from build123d import *

# Parameters (mm, degrees)
CROQUIS1_W              = 10
CROQUIS1_H              = 12.25
SALIENTE_EXTRUIR1_DEPTH = 6.5
CROQUIS3_R              = 1
CROQUIS3_W              = 12.25
CROQUIS3_H              = 3.5
CORTAR_EXTRUIR1_DEPTH   = 35.4


with BuildPart() as part:
    # Croquis1 → Saliente-Extruir1 (new body)
    with BuildSketch(Plane(origin=(0, 0, 0), x_dir=(1, 0, 0), z_dir=(0, 1, 0))):
        Polygon((-15.606807411, 13.619327476), (-15.606807411, 6.744327476), (-9.43180722, 6.744327476), (-9.43180722, -5.505672524), (-15.606807411, -5.505672524), (-15.606807411, -12.380672524), (17.093193352, -12.380672524), (17.093193352, -5.505672524), (10.918193161, -5.505672524), (10.918193161, 6.744327476), (17.093193352, 6.744327476), (17.093193352, 13.619327476), align=None)
        with Locations((0.743192971, 0.619327476)):
            Rectangle(CROQUIS1_W, CROQUIS1_H, mode=Mode.SUBTRACT)
    extrude(amount=SALIENTE_EXTRUIR1_DEPTH)

    # Croquis3 → Cortar-Extruir1 (cut)
    with BuildSketch(Plane.ZY.offset(15.606807411)):
        with Locations((-10.181827476, 3.25)):
            Circle(CROQUIS3_R)
        with Locations((8.943172524, 3.25)):
            Circle(CROQUIS3_R)
        with Locations((-0.619327476, 4.75)):
            Rectangle(CROQUIS3_W, CROQUIS3_H)
    extrude(amount=-CORTAR_EXTRUIR1_DEPTH, mode=Mode.SUBTRACT)


solid = part.part
CAD build for the part. Positions are in the model's coordinates, mm. A direction names the side the tool comes from. Give positions to 0.01 mm unless a question says otherwise; leave off trailing zeros. Write each loop counter-clockwise with the first axis right and the second up, starting at its lowest first coordinate (ties: lowest second). Pieces come first, ordered by that corner, then holes. Notation, with made-up numbers: (65, 3) -> (89, 3) arc R15 cw to (89, 21) -> close; hole circle Ø9 at (81.25, 71.5). An arc over 180 degrees is marked (long way). Return JSON: item names as keys, results as strings.
Item 1: Tool access for faces 5 (the flat face through (5.743, 1, -1)), 6 (the flat face through (1, 3, -6.744)), 7 (the flat face through (-7, 3, -1)), 8 (the flat face through (10.918, 1, -1)), 9 (the flat face through (-9.432, 1, -1)): list every direction of +Z, -Z, +X, -X, +Y, -Y with a clear straight run to the whole face (end or side of a thin tool).
Answer below:
{"face 5": "+Y, -Y", "face 6": "+Y", "face 7": "+X, -X, +Y", "face 8": "+X, +Y, -Y", "face 9": "-X, +Y, -Y"}
Item 2: Band-saw the part on A-A (x = 0.5). List the corners of the cut face in (y, z).
Answer below:
{"outline": "(0, -13.62) -> (6.5, -13.62) -> (6.5, -6.74) -> (0, -6.74) -> close; (0, 5.51) -> (6.5, 5.51) -> (6.5, 12.38) -> (0, 12.38) -> close; hole circle Ø2 at (3.25, -10.18); hole circle Ø2 at (3.25, 8.94)"}
Item 3: Drop flat-ended pins along their axis: pin 1 (2.5 mm diameter, centred on x = -7, z = -3, fed in from +Y); pin 2 (1.5 mm diameter, centred on y = 1, z = -3, fed in from +X); pin 3 (0.9 mm diameter, centred on y = 2, z = -0.5, fed in from -X). Give the stop position or say it passes through.
Answer below:
{"pin 1": "stops at y = 3", "pin 2": "stops at x = 10.92", "pin 3": "stops at x = -9.43"}
Item 4: Two-plate mould, pull along X, no slides. Class faces 1 (the flat face through (17.093, 2, -9)), 2 (the flat face through (-4.257, 1, -1)), 3 (the flat face through (-15.607, 2, 8)), 4 (the flat face through (1, 6.5, -10)): +X half, -X half, draft (parallel to the pull), parting line (faces both ways), or undercut.
Answer below:
{"face 1": "+X half", "face 2": "undercut", "face 3": "-X half", "face 4": "draft"}
Item 5: Band-saw the part on B-B (y = 6). List the corners of the cut face in (x, z).
Answer below:
{"outline": "(-15.61, -13.62) -> (17.09, -13.62) -> (17.09, -6.74) -> (-15.61, -6.74) -> close; (-15.61, 5.51) -> (17.09, 5.51) -> (17.09, 12.38) -> (-15.61, 12.38) -> close"}
Item 6: Drill centre lines: probe 1 along X at (y, z) = (2.25, 5.25); probe 2 along Z at (x, y) = (-13, 2); probe 3 along Y at (x, z) = (-1, 9). Where is each one in solid material? Low to high.
Answer below:
{"probe 1": "x = -9.43 to -4.26, 5.74 to 10.92", "probe 2": "z = -13.62 to -6.74, 5.51 to 12.38", "probe 3": "y = 0 to 2.25, 4.25 to 6.5"}
Item 7: Band-saw the part on C-C (z = 4.5). List the corners of the cut face in (x, y).
Answer below:
{"outline": "(-9.43, 0) -> (-4.26, 0) -> (-4.26, 3) -> (-9.43, 3) -> close; (5.74, 0) -> (10.92, 0) -> (10.92, 3) -> (5.74, 3) -> close"}
